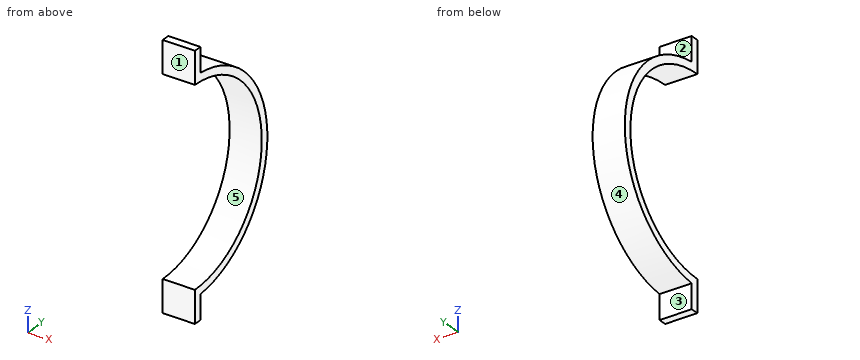
```python
from build123d import *

# Parameters (mm, degrees)
BOSS_EXTRUDE1_DEPTH = 10


with BuildPart() as part:
    # Sketch1 → Boss-Extrude1 (new body)
    with BuildSketch(Plane(origin=(0, 0, 0), x_dir=(0, 0, -1), z_dir=(1, 0, 0))):
        with BuildLine():
            Line((-30, 0), (-40, 0))
            Line((-40, 0), (-40, 2.5))
            Line((-40, 2.5), (-32.403703492, 2.5))
            ThreePointArc((-32.403703492, 2.5), (0, 32.5), (32.403703492, 2.5))
            Line((32.403703492, 2.5), (40, 2.5))
            Line((40, 2.5), (40, 0))
            Line((40, 0), (30, 0))
            ThreePointArc((30, 0), (0, 30), (-30, 0))
        make_face()
    extrude(amount=BOSS_EXTRUDE1_DEPTH)


solid = part.part
```
Input: part model. Units: mm. Frame: model coordinates. Face numbers are marked on the shaded views. A direction names the side the tool comes from. Coordinates: 2 decimals unless noted, no trailing zeros. Loops run counter-clockwise (first coordinate to the right, second up) from the corner with the lowest first, then second, coordinate; pieces in that order, holes last.
Q1. Contact query for flat-ended pins moving along their axis: pin 1 (6 mm diameter, centred on x = 7, z = -17, fed in from +Y); pin 2 (4 mm diameter, centred on x = 3, z = -34.5, fed in from +Y); pin 3 (2 mm diameter, centred on x = 7, z = -23.5, fed in from +Y). Output: stop coordinate, or through.
Results are:
pin 1: stops at y = 29.33
pin 2: stops at y = 2.5
pin 3: stops at y = 23.45
Q2. Section D-D, the plane y = 4. Return the cut outline in (x, z), and give its area (3 significant figures).
Results are:
outline: (0, -32.25) - (10, -32.25) - (10, -29.73) - (0, -29.73) - close; (0, 29.73) - (10, 29.73) - (10, 32.25) - (0, 32.25) - close
area: 50.4 mm2
Q3. Set-up query: the marked faces 1 and 2. Return all of +Z, -Z, +X, -X, +Y, -Y with unobstructed straight access to the full face (end or side cutting, diameter ignored); none if empty.
Results are:
face 1: +Z, -Z, +X, -X, -Y
face 2: +Z, +X, -X, +Y
Q4. Mould query, pull axis Z, two halves, no side actions, for the marked faces 3, 4 and 5. Classes: +Z half, -Z half, draft (parallel to the pull), parting line (faces both ways), or undercut.
Results are:
face 3: draft
face 4: parting line
face 5: undercut
Q5. Section A-A, the plane y = 9. Return the cut outline in (x, z), and give its area (3 significant figures).
Results are:
outline: (0, -31.23) - (10, -31.23) - (10, -28.62) - (0, -28.62) - close; (0, 28.62) - (10, 28.62) - (10, 31.23) - (0, 31.23) - close
area: 52.2 mm2
Q6. Section B-B, the plane x = 3.25. Return the cut outline in (y, z), and give its area (3 significant figures).
Results are:
outline: (0, -40) - (2.5, -40) - (2.5, -32.4) arc R32.5 ccw to (2.5, 32.4) - (2.5, 40) - (0, 40) - (0, 30) arc R30 cw to (0, -30) - close
area: 283 mm2
Q7. Section C-C, the plane z = 0. Return the cut outline in (x, y), and give its area (3 significant figures).
Results are:
outline: (0, 30) - (10, 30) - (10, 32.5) - (0, 32.5) - close
area: 25.0 mm2
Q8. Line query: line 1 along Y through (x, z) = (8.25, 36); line 2 along Z through (x, y) = (4, 15); line 3 along Z through (x, y) = (3.5, 8). Output: solid intervals per line, ascending.
Results are:
line 1: y = 0 to 2.5
line 2: z = -28.83 to -25.98, 25.98 to 28.83
line 3: z = -31.5 to -28.91, 28.91 to 31.5
